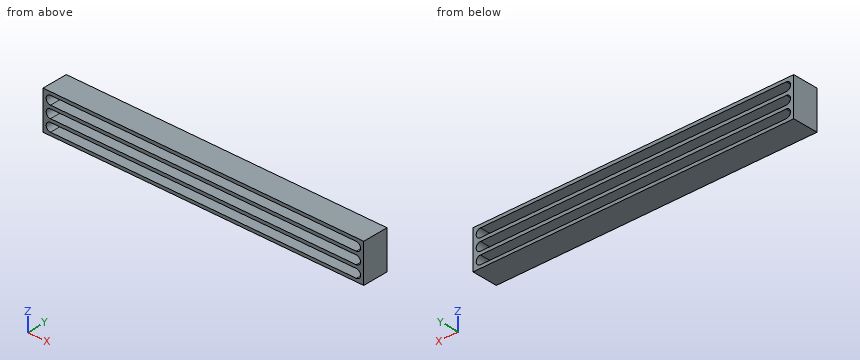
```python
from build123d import *

# Parameters (mm, degrees)
SKETCH1_W           = 635
SKETCH1_H           = 76.2
BOSS_EXTRUDE1_DEPTH = 50.8


with BuildPart() as part:
    # Sketch1 → Boss-Extrude1 (new body)
    with BuildSketch(Plane(origin=(0, 0, 0), x_dir=(1, 0, 0), z_dir=(0, 1, 0))):
        Rectangle(SKETCH1_W, SKETCH1_H)
        with BuildLine():
            Line((302.683333333, -8.382), (-302.683333333, -8.382))
            ThreePointArc((-302.683333333, -8.382), (-311.15, 0.084666667), (-302.683333333, 8.551333333))
            Line((-302.683333333, 8.551333333), (302.683333333, 8.551333333))
            ThreePointArc((302.683333333, 8.551333333), (311.15, 0.084666667), (302.683333333, -8.382))
        make_face(mode=Mode.SUBTRACT)
        with BuildLine():
            Line((302.683333333, -31.75), (-302.683333333, -31.75))
            ThreePointArc((-302.683333333, -31.75), (-311.15, -23.283333333), (-302.683333333, -14.816666667))
            Line((-302.683333333, -14.816666667), (302.683333333, -14.816666667))
            ThreePointArc((302.683333333, -14.816666667), (311.15, -23.283333333), (302.683333333, -31.75))
        make_face(mode=Mode.SUBTRACT)
        with BuildLine():
            Line((302.683333333, 14.986), (-302.683333333, 14.986))
            ThreePointArc((-302.683333333, 14.986), (-311.15, 23.452666667), (-302.683333333, 31.919333333))
            Line((-302.683333333, 31.919333333), (302.683333333, 31.919333333))
            ThreePointArc((302.683333333, 31.919333333), (311.15, 23.452666667), (302.683333333, 14.986))
        make_face(mode=Mode.SUBTRACT)
    extrude(amount=-BOSS_EXTRUDE1_DEPTH)


solid = part.part
```
Source: CAD feature listing. Evaluate the final solid. Frame: model axes, mm. Coordinates: 2 decimals unless noted, no trailing zeros. Loops run counter-clockwise (first coordinate to the right, second up) from the corner with the lowest first, then second, coordinate; pieces in that order, holes last. Notation, with made-up numbers: M -0.75,57 L 55.25,57 A31 ccw 55.25,93 Z; hole C 40,72.25 d4. An arc over 180 degrees is marked long. Use a Markdown table: item, result. Add a question column.
Q1. First-contact query: pin 1 (5 mm diameter, centred on x = -145.5, z = 5.5, fed in from +Y). Flat tip, straight axial feed; report the tip coordinate or a pass-through.
Q2. Section query B-B, the plane y = -13. Return loops of the section in (x, z), and give its area (3 significant figures).
Q3. Section query A-A, the plane x = 188. Return loops of the section in (y, z).
Q4. Material intervals for L1, parallel to Z at x = 53, y = -33.5; L2, parallel to X at y = -45.5, z = -22; L3, parallel to X at y = -17.5, z = -0.5, sorted ascending.
Result:
| question | item | result |
|---|---|---|
| 1 | pin 1 | passes through |
| 2 | outline | M -317.5,-38.1 L 317.5,-38.1 L 317.5,38.1 L -317.5,38.1 Z; hole M -302.68,-31.92 L 302.68,-31.92 A8.47 ccw 302.68,-14.99 L -302.68,-14.99 A8.47 ccw Z; hole M -302.68,-8.55 L 302.68,-8.55 A8.47 ccw 302.68,8.38 L -302.68,8.38 A8.47 ccw Z; hole M -302.68,14.82 L 302.68,14.82 A8.47 ccw 302.68,31.75 L -302.68,31.75 A8.47 ccw Z |
| 2 | area | 17,000 mm2 |
| 3 | outline | M -50.8,-38.1 L 0,-38.1 L 0,-31.92 L -50.8,-31.92 Z; M -50.8,-14.99 L 0,-14.99 L 0,-8.55 L -50.8,-8.55 Z; M -50.8,8.38 L 0,8.38 L 0,14.82 L -50.8,14.82 Z; M -50.8,31.75 L 0,31.75 L 0,38.1 L -50.8,38.1 Z |
| 4 | L1 | z = -38.1 to -31.92, -14.99 to -8.55, 8.38 to 14.82, 31.75 to 38.1 |
| 4 | L2 | x = -317.5 to -311.02, 311.02 to 317.5 |
| 4 | L3 | x = -317.5 to -311.14, 311.14 to 317.5 |
